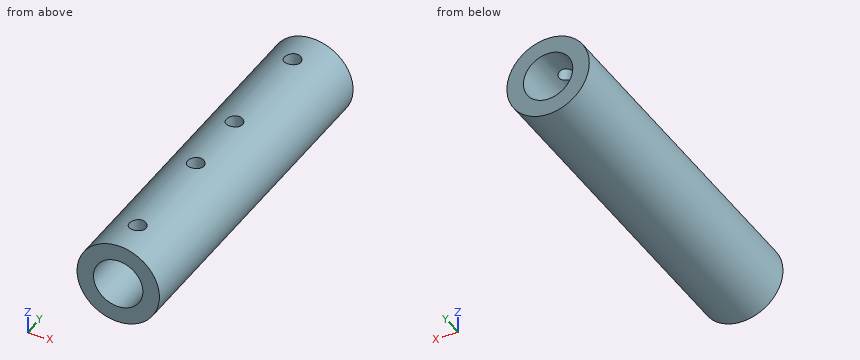
Autodesk Inventor part; units mm, degrees
sketch "Sketch1" plane through (0, 0, 0) normal (0, 1, 0) x (-1, 0, 0)
  circle A0 centre (0, 0) radius 2.1
  circle A1 centre (0, 0) radius 3.5
  line L0 (0, -2.1) -> (0, -3.5)
  dimension "d0" = 4.2
  dimension "d1" = 7
extrude "Extrusion1" add sketch "Sketch1" along normal blind 15
sketch "Sketch2" plane through (0, 0, 0) normal (0, 0, 1) x (1, 0, 0)
  point P0 (0, 0)
  point P1 (0.0001, 11.9963)
hole "Hole1" at (0.0001, 11.9963, 0) direction (0, 0, 1) diameter 1.4 depth 4.8 tip angle 118
ref_plane "Work Plane1" through (0, 7.5, 0) normal (0, 1, 0) x (1, 0, 0)
mirror "Mirror1" about plane through (0, 7.5, 0) normal (0, 1, 0) of "Hole1"
mirror "Mirror2" about plane through (0, 0, 0) normal (0, 1, 0) of "Extrusion1"
mirror "Mirror3" about plane through (0, 0, 0) normal (0, 1, 0) of "Hole1", "Mirror1"
properties part number "Colletto 3mm_3DPrint"
Check sheet for the modelled part. Datum: model origin and axes. Units: mm. Round coordinates to 2 decimals unless told otherwise and drop trailing zeros. Loops run counter-clockwise (first coordinate to the right, second up) from the corner with the lowest first, then second, coordinate; pieces in that order, holes last. Notation, with made-up numbers: M 60,-19.75 L 99,-19.75 A18 ccw 99,9.25 Z; hole C 74,4.5 d11. An arc over 180 degrees is marked long. Answer as a JSON object with one key per item and string values.
1. Section check A-A (z = 0). Record the boundary of the cut face in (x, y), plus the area to 3 significant figures.
Reply:
{"outline": "M -3.5,-15 L -2.1,-15 L -2.1,15 L -3.5,15 Z; M 2.1,-15 L 3.5,-15 L 3.5,15 L 2.1,15 Z", "area": "84.0 mm²"}
2. Scan lines: line 1 (Z direction, x = 0, y = 6.5); line 2 (Z direction, x = -1.5, y = 6.5). Record each from-to range of solid material in increasing order.
Reply:
{"line 1": "z = -3.5 to -2.1, 2.1 to 3.5", "line 2": "z = -3.16 to -1.47, 1.47 to 3.16"}
3. Gauge pin test, flat ends, axial feed: P1, Ø2.5, axis at x = 0, z = 0, coming from the -Y side; P2, Ø1.1, axis at x = 0, y = 12, coming from the +Z side; P3, Ø3, axis at y = -8, z = -2, coming from the +X side. Record the tip position at first contact, or that the pin passes through.
Reply:
{"P1": "passes through", "P2": "stops at z = -2.03", "P3": "stops at x = 3.46"}
4. Section check C-C (z = 2.5). Record the boundary of the cut face in (x, y), plus the area to 3 significant figures.
Reply:
{"outline": "M -2.45,-15 L 2.45,-15 L 2.45,15 L -2.45,15 Z; hole C 0,-12 d1.4; hole C 0,-3 d1.4; hole C 0,3 d1.4; hole C 0,12 d1.4", "area": "141 mm²"}
5. Section check B-B (x = -1.75). Record the boundary of the cut face in (y, z), plus the area to 3 significant figures.
Reply:
{"outline": "M -15,-3.03 L 15,-3.03 L 15,-1.16 L -15,-1.16 Z; M -15,1.16 L 15,1.16 L 15,3.03 L -15,3.03 Z", "area": "112 mm²"}
6. Section check D-D (y = -7). Record the boundary of the cut face in (x, z).
Reply:
{"outline": "C 0,0 d7; hole C 0,0 d4.2"}
